```python
from build123d import *

# Parameters (mm, degrees)
SKETCH_1_W          = 193
SKETCH_1_H          = 110.8
EXTRUDE_1_DEPTH     = 0.75
FILLET_1_R          = 8.4
SKETCH_2_W          = 166.3
SKETCH_2_H          = 100.7
EXTRUDE_2_DEPTH     = 5.6
SKETCH_3_W          = 6
SKETCH_3_H          = 8
EXTRUDE_3_DEPTH     = 2.34
CHAMFER_1_SIZE      = 2.34
SKETCH_4_R          = 1.35
CUT_EXTRUDE_1_DEPTH = 2.34
SKETCH_5_W          = 7.8
SKETCH_5_H          = 7.8
EXTRUDE_4_DEPTH     = 2.34
SKETCH_6_W          = 65
SKETCH_6_H          = 56
EXTRUDE_5_DEPTH     = 1.2
FILLET_2_R          = 2.5
SKETCH_7_R          = 1.25
CUT_EXTRUDE_2_DEPTH = 0.6


with BuildPart() as part:
    # 草图1 → 凸台-拉伸1 (new body)
    with BuildSketch(Plane.XY):
        Rectangle(SKETCH_1_W, SKETCH_1_H)
    extrude(amount=EXTRUDE_1_DEPTH)

    # 圆角1
    fillet_1_edges = [part.edges().sort_by_distance(p)[0] for p in [
        (96.5, -55.4, 0.375),
        (-96.5, -55.4, 0.375),
        (-96.5, 55.4, 0.375),
        (96.5, 55.4, 0.375),
    ]]
    fillet(fillet_1_edges, radius=FILLET_1_R)

    # 草图2 → 凸台-拉伸2 (add)
    with BuildSketch(Plane(origin=(0, 0, 0), x_dir=(-1, 0, 0), z_dir=(0, 0, -1))):
        Rectangle(SKETCH_2_W, SKETCH_2_H)
    extrude(amount=EXTRUDE_2_DEPTH)

    # 草图3 → 凸台-拉伸3 (add)
    with BuildSketch(Plane(origin=(0, 0, -5.6), x_dir=(-1, 0, 0), z_dir=(0, 0, -1))):
        with Locations((-63, 34.1)):
            Rectangle(SKETCH_3_W, SKETCH_3_H)
        with Locations((-63, -31.9)):
            Rectangle(SKETCH_3_W, SKETCH_3_H)
        with Locations((63, 34.1)):
            Rectangle(SKETCH_3_W, SKETCH_3_H)
        with Locations((63, -31.9)):
            Rectangle(SKETCH_3_W, SKETCH_3_H)
    extrude(amount=EXTRUDE_3_DEPTH)

    # 倒角1
    chamfer_1_edges = [part.edges().sort_by_distance(p)[0] for p in [
        (66, -31.9, -5.6),
        (60, -31.9, -5.6),
        (-66, -31.9, -5.6),
        (-60, -31.9, -5.6),
        (-60, 34.1, -5.6),
        (-66, 34.1, -5.6),
        (60, 34.1, -5.6),
        (66, 34.1, -5.6),
    ]]
    chamfer(chamfer_1_edges, length=CHAMFER_1_SIZE - 0.0001)  # a hair under: the kernel refuses the full size

    # 草图4 → 切除-拉伸1 (cut)
    with BuildSketch(Plane(origin=(0, 0, -7.94), x_dir=(-1, 0, 0), z_dir=(0, 0, -1))):
        with Locations((-63, 34.1)):
            Circle(SKETCH_4_R)
        with Locations((-63, -31.9)):
            Circle(SKETCH_4_R)
        with Locations((63, -31.9)):
            Circle(SKETCH_4_R)
        with Locations((63, 34.1)):
            Circle(SKETCH_4_R)
    extrude(amount=-CUT_EXTRUDE_1_DEPTH, mode=Mode.SUBTRACT)

    # 草图5 → 凸台-拉伸4 (add)
    with BuildSketch(Plane(origin=(0, 0, -5.6), x_dir=(-1, 0, 0), z_dir=(0, 0, -1))):
        with Locations((-35.8, 31.4)):
            Rectangle(SKETCH_5_W, SKETCH_5_H)
        with Locations((22.2, 31.4)):
            Rectangle(SKETCH_5_W, SKETCH_5_H)
        with Locations((-35.8, -17.6)):
            Rectangle(SKETCH_5_W, SKETCH_5_H)
        with Locations((22.2, -17.6)):
            Rectangle(SKETCH_5_W, SKETCH_5_H)
    extrude(amount=EXTRUDE_4_DEPTH)

    # 草图6 → 凸台-拉伸5 (add)
    with BuildSketch(Plane(origin=(0, 0, -7.94), x_dir=(-1, 0, 0), z_dir=(0, 0, -1))):
        with Locations((-6.9, 7)):
            Rectangle(SKETCH_6_W, SKETCH_6_H)
    extrude(amount=EXTRUDE_5_DEPTH)

    # 圆角2
    fillet_2_edges = [part.edges().sort_by_distance(p)[0] for p in [
        (-25.6, -21, -8.54),
        (-25.6, 35, -8.54),
        (39.4, 35, -8.54),
        (39.4, -21, -8.54),
    ]]
    fillet(fillet_2_edges, radius=FILLET_2_R)

    # 草图7 → 切除-拉伸2 (cut)
    with BuildSketch(Plane(origin=(0, 0, -9.14), x_dir=(-1, 0, 0), z_dir=(0, 0, -1))):
        with Locations((-35.8, 31.4)):
            Circle(SKETCH_7_R)
        with Locations((22.2, 31.4)):
            Circle(SKETCH_7_R)
        with Locations((-35.8, -17.6)):
            Circle(SKETCH_7_R)
        with Locations((22.2, -17.6)):
            Circle(SKETCH_7_R)
    extrude(amount=-CUT_EXTRUDE_2_DEPTH, mode=Mode.SUBTRACT)


solid = part.part
```
Geometry check sheet. Reference: the model listing, model coordinates, mm. A direction names the side the tool comes from. Round coordinates to 2 decimals unless told otherwise and drop trailing zeros. Write each loop counter-clockwise with the first axis right and the second up, starting at its lowest first coordinate (ties: lowest second). Pieces come first, ordered by that corner, then holes. Notation, with made-up numbers: (52, 35) -> (64, 35) arc R11 cw to (64, 40) -> close; hole circle Ø6 at (-39.75, 85.5). An arc over 180 degrees is marked (long way). Put each result on its own line as item: value.
1) Cross-section at C-C, the plane y = -42. Enter the section's corners in (x, z).
Recorded:
outline: (-96.5, 0) -> (-83.15, 0) -> (-83.15, -5.6) -> (83.15, -5.6) -> (83.15, 0) -> (96.5, 0) -> (96.5, 0.75) -> (-96.5, 0.75) -> close
2) Thickness scan on probe 1 along Y at (x, z) = (-22.2, -8.65); probe 2 along Y at (x, z) = (63, -6.25); probe 3 along Z at (x, y) = (-13, 23). Record the ranges inside material, lowest first. Write a range as from..to.
Recorded:
probe 1: y = -21..-18.85, -16.35..30.15, 32.65..35
probe 2: y = -35.9..-33.25, -30.55..-27.9, 30.1..32.75, 35.45..38.1
probe 3: z = -9.14..-7.94, -5.6..0.75
3) Cross-section at B-B, the plane x = 76.5. Enter the section's corners in (y, z).
Recorded:
outline: (-55.4, 0) -> (-50.35, 0) -> (-50.35, -5.6) -> (50.35, -5.6) -> (50.35, 0) -> (55.4, 0) -> (55.4, 0.75) -> (-55.4, 0.75) -> close
4) Cross-section at A-A, the plane y = 22. Enter the section's corners in (x, z), plus the area to 3 significant figures.
Recorded:
outline: (-96.5, 0) -> (-83.15, 0) -> (-83.15, -5.6) -> (83.15, -5.6) -> (83.15, 0) -> (96.5, 0) -> (96.5, 0.75) -> (-96.5, 0.75) -> close; (-25.6, -9.14) -> (39.4, -9.14) -> (39.4, -7.94) -> (-25.6, -7.94) -> close
area: 1,150 mm2
5) Access from +Z, -Z, +X, -X, +Y, -Y to the whole of each face (thin tool, end or side, straight path). Record for faces 4 (the face through (0, -53, 0)), 5 (the face through (38, -21, -7.94)), 6 (the face through (-83.15, -1, -3)).
Recorded:
face 4: -Z
face 5: -Z, +X, -Y
face 6: -Z, -X, +Y, -Y
6) Depth check by flat-ended pin: P1, Ø0.7, axis at x = 63, z = -7, coming from the -Y side; P2, Ø1.5, axis at x = 46, y = -10, coming from the -Z side; P3, Ø1.9, axis at x = -22.5, z = -7, coming from the +Y side. Enter the tip coordinate at first touch or a pass-through.
Recorded:
P1: stops at y = -35.9
P2: stops at z = -5.6
P3: stops at y = 35.3
7) Release check for a two-part mould opening along X. For faces 1 (the face through (1, -50.35, -3)), 2 (the face through (93.974, -53.005, 0.38)), 3 (the face through (7, 7, -7.94)) record: pulls with the +X half, pulls with the -X half, needs draft (parallel to the pull), parting line crosses it, or undercut.
Recorded:
face 1: needs draft
face 2: pulls with the +X half
face 3: undercut
8) Cross-section at D-D, the plane z = -2.25. Enter the section's corners in (x, y).
Recorded:
outline: (-83.15, -50.35) -> (83.15, -50.35) -> (83.15, 50.35) -> (-83.15, 50.35) -> close
